Autodesk Inventor part; units mm, degrees
ref_plane "YZ Plane" through (0, 0, 0) normal (1, 0, 0) x (0, 1, 0)
ref_plane "XZ Plane" through (0, 0, 0) normal (0, 1, 0) x (-1, 0, 0)
ref_plane "XY Plane" through (0, 0, 0) normal (0, 0, 1) x (1, 0, 0)
sketch "Sketch1" plane through (0, 0, 0) normal (0, 1, 0) x (-1, 0, 0)
  line L0 (0, 0) -> (-6.35, 0)
  line L1 (-6.35, 0) -> (-6.35, -80)
  line L2 (-6.35, -80) -> (0, -80)
  line L3 (0, -80) -> (0, 0)
  dimension "d0" = 6.35
  dimension "d1" = 80
extrude "Extrusion1" add sketch "Sketch1" along normal blind 6.35
sketch "Sketch2" plane through (0, 6.35, 0) normal (0, 1, 0) x (1, 0, 0)
  line L0 (0, 0) -> (6.35, 0)
  line L1 (6.35, 0) -> (0, 6.35)
  line L2 (0, 80) -> (0, 0)
  line L3 (6.35, 0) -> (15.3303, 0) construction
  line L4 (0, 6.35) -> (0, 0)
  line L5 (0, 0) -> (6.35, 0)
  dimension "d4" = 135
extrude "Extrusion2" cut sketch "Sketch2" against normal blind 10
sketch "Sketch3" plane through (0, 6.35, 0) normal (0, 1, 0) x (1, 0, 0)
  line L0 (6.35, 80) -> (0, 73.65)
  line L1 (6.35, 80) -> (15.3303, 80) construction
  line L2 (0, 73.65) -> (0, 80)
  line L3 (6.35, 0) -> (6.35, 80)
  line L4 (6.35, 80) -> (0, 80)
  line L5 (0, 80) -> (6.35, 80)
  point P0 (0, 0)
  dimension "d7" = 135
extrude "Extrusion3" cut sketch "Sketch3" against normal blind 10
properties part number "5"
Work out the finished part from the listing and answer in its coordinate system (mm). Give positions to 0.01 mm unless a question says otherwise; leave off trailing zeros. Loops run counter-clockwise (first coordinate to the right, second up) from the corner with the lowest first, then second, coordinate; pieces in that order, holes last. Notation, with made-up numbers: (55, 56.25) -> (113, 56.25) arc R27 ccw to (113, 91.25) -> close; hole circle Ø7 at (84, -21.75). An arc over 180 degrees is marked (long way). Use a Markdown table: item, result. Add a question column.
1) The part is cut by section A-A, the plane x = 4.25. Determine the outline of the cut face in (y, z).
2) Consider line 1 along X through (y, z) = (4.75, -4); line 2 along Z through (x, y) = (0.75, 0.75); line 3 along Z through (x, y) = (1, 4.75). Determine where each line is inside the solid, lowest interval first.
3) The part is cut by section B-B, the plane y = 2.75. Determine the outline of the cut face in (x, z).
Reported:
| question | item | result |
|---|---|---|
| 1 | outline | (0, -77.9) -> (6.35, -77.9) -> (6.35, -2.1) -> (0, -2.1) -> close |
| 2 | line 1 | x = 2.35 to 6.35 |
| 2 | line 2 | z = -74.4 to -5.6 |
| 2 | line 3 | z = -74.65 to -5.35 |
| 3 | outline | (0, -73.65) -> (6.35, -80) -> (6.35, 0) -> (0, -6.35) -> close |
